```python
from build123d import *

# Parameters (mm, degrees)
SKETCH_1_W          = 147
SKETCH_1_H          = 25
EXTRUDE_1_DEPTH     = 1.5
CUT_EXTRUDE_1_DEPTH = 2.5
CUT_EXTRUDE_2_DEPTH = 10
FILLET_2_R          = 0.5
SKETCH_4_W          = 10
SKETCH_4_H          = 25
EXTRUDE_2_DEPTH     = 1.5
FILLET_3_R          = 0.5
SKETCH_5_R          = 1.75
CUT_EXTRUDE_3_DEPTH = 2.5
CUT_EXTRUDE_4_DEPTH = 2.5


with BuildPart() as part:
    # 草图1 → 凸台-拉伸1 (new body)
    with BuildSketch(Plane(origin=(0, 0, 0), x_dir=(1, 0, 0), z_dir=(0, 1, 0))):
        Rectangle(SKETCH_1_W, SKETCH_1_H)
    extrude(amount=EXTRUDE_1_DEPTH)

    # 草图2 → 切除-拉伸1 (cut, through all)
    with BuildSketch(Plane.XZ):
        Polygon((10, 2.5), (-10, 2.5), (-22.5, 12.5), (22.5, 12.5), align=None)
    extrude(amount=-CUT_EXTRUDE_1_DEPTH, mode=Mode.SUBTRACT)

    # 草图3 → 切除-拉伸2 (cut)
    with BuildSketch(Plane.XZ):
        Polygon((-4.802343178, -9.5), (-16.052343178, -0.5), (-28.552343178, 9.5), (-33.552343178, 9.5), (-21.052343178, -0.5), (-9.802343178, -9.5), align=None)
        Polygon((-26.052343178, -0.5), (-38.552343178, 9.5), (-43.552343178, 9.5), (-31.052343178, -0.5), (-19.802343178, -9.5), (-14.802343178, -9.5), align=None)
        Polygon((-36.052343178, -0.5), (-48.552343178, 9.5), (-53.552343178, 9.5), (-41.052343178, -0.5), (-29.802343178, -9.5), (-24.802343178, -9.5), align=None)
        Polygon((-46.052343178, -0.5), (-58.552343178, 9.5), (-63.552343178, 9.5), (-51.052343178, -0.5), (-39.802343178, -9.5), (-34.802343178, -9.5), align=None)
        Polygon((-56.052343178, -0.5), (-68.552343178, 9.5), (-70.5, 9.5), (-70.5, 7.058125458), (-61.052343178, -0.5), (-49.802343178, -9.5), (-44.802343178, -9.5), align=None)
        Polygon((-59.802343178, -9.5), (-54.802343178, -9.5), (-66.052343178, -0.5), (-70.5, 3.058125458), (-70.5, -0.941874542), align=None)
        Polygon((-70.5, -9.5), (-64.802343178, -9.5), (-70.5, -4.941874542), align=None)
    cut_extrude_2 = extrude(amount=-CUT_EXTRUDE_2_DEPTH, mode=Mode.SUBTRACT)

    # 镜向3: 切除-拉伸2 across plane
    add(cut_extrude_2.mirror(Plane(origin=(0, 0, 0), x_dir=(0, 0, 1), z_dir=(1, 0, 0))), mode=Mode.SUBTRACT)

    # 圆角2
    fillet_2_edges = [part.edges().sort_by_distance(p)[0] for p in [
        (-70.5, 0.75, -0.941874542),
        (-70.5, 0.75, 3.058125458),
        (-54.802343178, 0.75, -9.5),
        (-59.802343178, 0.75, -9.5),
        (-9.802343178, 0.75, -9.5),
        (-33.552343178, 0.75, 9.5),
        (-28.552343178, 0.75, 9.5),
        (-4.802343178, 0.75, -9.5),
        (22.5, 0.75, 12.5),
        (10, 0.75, 2.5),
        (-10, 0.75, 2.5),
        (-22.5, 0.75, 12.5),
        (63.552343178, 0.75, 9.5),
        (39.802343178, 0.75, -9.5),
        (34.802343178, 0.75, -9.5),
        (58.552343178, 0.75, 9.5),
        (70.5, 0.75, 7.058125458),
        (49.802343178, 0.75, -9.5),
        (44.802343178, 0.75, -9.5),
        (68.552343178, 0.75, 9.5),
        (70.5, 0.75, 9.5),
        (43.552343178, 0.75, 9.5),
        (19.802343178, 0.75, -9.5),
        (14.802343178, 0.75, -9.5),
        (38.552343178, 0.75, 9.5),
        (53.552343178, 0.75, 9.5),
        (29.802343178, 0.75, -9.5),
        (24.802343178, 0.75, -9.5),
        (48.552343178, 0.75, 9.5),
        (64.802343178, 0.75, -9.5),
        (70.5, 0.75, -4.941874542),
        (70.5, 0.75, -9.5),
        (70.5, 0.75, 3.058125458),
        (70.5, 0.75, -0.941874542),
        (59.802343178, 0.75, -9.5),
        (54.802343178, 0.75, -9.5),
        (33.552343178, 0.75, 9.5),
        (9.802343178, 0.75, -9.5),
        (4.802343178, 0.75, -9.5),
        (28.552343178, 0.75, 9.5),
        (-39.802343178, 0.75, -9.5),
        (-63.552343178, 0.75, 9.5),
        (-58.552343178, 0.75, 9.5),
        (-34.802343178, 0.75, -9.5),
        (-49.802343178, 0.75, -9.5),
        (-70.5, 0.75, 7.058125458),
        (-70.5, 0.75, 9.5),
        (-68.552343178, 0.75, 9.5),
        (-44.802343178, 0.75, -9.5),
        (73.5, 0.75, 12.5),
        (-19.802343178, 0.75, -9.5),
        (-73.5, 0.75, 12.5),
        (-43.552343178, 0.75, 9.5),
        (-38.552343178, 0.75, 9.5),
        (-14.802343178, 0.75, -9.5),
        (-73.5, 0.75, -12.5),
        (73.5, 0.75, -12.5),
        (-29.802343178, 0.75, -9.5),
        (-53.552343178, 0.75, 9.5),
        (-48.552343178, 0.75, 9.5),
        (-24.802343178, 0.75, -9.5),
        (-70.5, 0.75, -4.941874542),
        (-64.802343178, 0.75, -9.5),
        (-70.5, 0.75, -9.5),
    ]]
    fillet(fillet_2_edges, radius=FILLET_2_R)

    # 草图4 → 凸台-拉伸2 (add)
    with BuildSketch(Plane(origin=(0, 1.5, 0), x_dir=(1, 0, 0), z_dir=(0, 1, 0))):
        with Locations((68.5, 0)):
            Rectangle(SKETCH_4_W, SKETCH_4_H)
    extrude_2 = extrude(amount=-EXTRUDE_2_DEPTH)

    # 镜向4: 凸台-拉伸2 across plane
    add(extrude_2.mirror(Plane(origin=(0, 0, 0), x_dir=(0, 0, 1), z_dir=(1, 0, 0))))

    # 圆角3
    fillet_3_edges = [part.edges().sort_by_distance(p)[0] for p in [
        (63.5, 0.75, 5.458125458),
        (63.5, 0.75, -6.541874542),
        (63.5, 0.75, -2.541874542),
        (63.5, 0.75, 1.458125458),
        (-63.5, 0.75, 5.458125458),
        (-63.5, 0.75, -2.541874542),
        (-63.5, 0.75, 1.458125458),
        (-63.5, 0.75, -6.541874542),
    ]]
    fillet(fillet_3_edges, radius=FILLET_3_R)

    # 草图5 → 切除-拉伸3 (cut, through all)
    with BuildSketch(Plane.XZ):
        with Locations((-68.5, -0.5)):
            Circle(SKETCH_5_R)
        with Locations((68.5, -0.5)):
            Circle(SKETCH_5_R)
    extrude(amount=-CUT_EXTRUDE_3_DEPTH, mode=Mode.SUBTRACT)

    # 草图6 → 切除-拉伸4 (cut, through all)
    with BuildSketch(Plane(origin=(0, 1.5, 0), x_dir=(1, 0, 0), z_dir=(0, 1, 0))):
        with BuildLine():
            Line((3, 8.5), (3, 7.5))
            ThreePointArc((3, 7.5), (0, 4.5), (-3, 7.5))
            Line((-3, 7.5), (-3, 8.5))
            ThreePointArc((-3, 8.5), (0, 11.5), (3, 8.5))
        make_face()
    extrude(amount=-CUT_EXTRUDE_4_DEPTH, mode=Mode.SUBTRACT)


solid = part.part
```
The listing builds one solid part. Answer for the finished solid, in the listing's coordinates (mm). A direction names the side the tool comes from. Give positions to 0.01 mm unless a question says otherwise; leave off trailing zeros. Order: outer loops, then holes, each group sorted by start corner. A loop starts at its lowest first (then second) coordinate and runs counter-clockwise, first axis right, second up. Notation, with made-up numbers: (11.5, 27) -> (34.5, 27) arc R21 ccw to (34.5, 41) -> close; hole circle Ø1 at (80.25, 4.5). An arc over 180 degrees is marked (long way). Answer as a JSON object with one key per item and string values. Group by question number.
Item 1: Consider L1, parallel to Z at x = 68.5, y = 0.7; L2, parallel to Z at x = 26, y = 0.85; L3, parallel to Z at x = 34.5, y = 1.15. Determine where each line is inside the solid, lowest interval first. Write a range as from..to.
Item 2: The part is cut by section C-C on y = 1.05. Give the number of separate pieces and of enclosed holes in the cut face, and give its area (3 significant figures).
Item 3: The part is cut by section B-B on x = 0. Write down the section's boundary in (y, z), and give its area (3 significant figures).
Item 4: The part is cut by section A-A on x = 68.5. Write down the section's boundary in (y, z), and give its area (4 significant figures).
Item 5: A tool of negligible diameter and unlimited length cuts with its end or side. For faces 1 (the flat face through (-41.3, 0.7, -0.3)), 2 (the flat face through (-16.16, 0.74, 7.43)), from which of +Z, -Z, +X, -X, +Y, -Y can it reach the whole face along a straight path? Write none if from no direction.
Item 6: A flat-ended cylindrical pin translates along its axis: pin 1 (6 mm diameter, centred on x = 35, z = -7, fed in from -Y). Find the tip coordinate at first contact, or state that the pin passes through.
Result set:
{
 "1": {"L1": "-12.5..-2.25, 1.25..12.5", "L2": "-12.5..-9.45, -8.54..-4.54, -0.54..3.46, 7.46..12.5", "L3": "-12.5..-5.74, -1.74..2.26, 6.26..12.5"},
 "2": {"separate pieces": "1", "enclosed holes": "15", "area": "2,370 mm²"},
 "3": {"outline": "(0, -12.5) -> (1.5, -12.5) -> (1.5, -11.5) -> (0, -11.5) -> close; (0, -4.5) -> (1.5, -4.5) -> (1.5, 2.5) -> (0, 2.5) -> close", "area": "12.0 mm²"},
 "4": {"outline": "(0, -12.5) -> (1.5, -12.5) -> (1.5, -2.25) -> (0, -2.25) -> close; (0, 1.25) -> (1.5, 1.25) -> (1.5, 12.5) -> (0, 12.5) -> close", "area": "32.25 mm²"},
 "5": {"face 1": "+Y, -Y", "face 2": "+Z, +Y, -Y"},
 "6": {"pin 1": "y = 0"}
}
